Read the model definition and answer for the solid it produces. Units are mm, in the model's axes. A direction names the side the tool comes from. Coordinates: 2 decimals unless noted, no trailing zeros. Loops run counter-clockwise (first coordinate to the right, second up) from the corner with the lowest first, then second, coordinate; pieces in that order, holes last. Notation, with made-up numbers: (35, 66.25) -> (93, 66.25) arc R25 ccw to (93, 93.25) -> close; hole circle Ø3 at (35.5, 22.5). An arc over 180 degrees is marked (long way). Answer as a JSON object with one key per item and string values. Group by question number.
Q1. Determine the mould class of faces 1 (the flat face through (0, 0, -1.5)), 2 (the conical face through (17.49, 5.51, 0.34)), 3 (the cylindrical face through (0.526, 2.007, 77.669)) for opening direction X: released by +X, released by -X, zero draft, split by the parting line, or undercut.
Q2. Straight lines are drawn through the part: line 1 along Z through (x, y) = (-5, 4); line 2 along X through (y, z) = (2, 76); line 3 along Y through (x, z) = (0, 16.5). For each, find the intervals that lie inside material, in ascending order. Write a range as [from, to].
Q3. For faces 4 (the cylindrical face through (-0.867, -3.905, 67.649)), 5 (the flat face through (0, 2.5, 79)), 6 (the flat face through (8, -8, 0)), 7 (the flat face through (0, 1.5, 76)), determine the directions among +Z, -Z, +X, -X, +Y, -Y from which every point of the face is accessible in a straight line to the end or side of a thin tool.
Q4. The part is cut by section B-B on z = 23. Write down the section's boundary in (x, y), and give its area (3 significant figures).
Q5. Each of these flat-tipped pins is pushed along its axis until it touches: P1, Ø1, axis at y = -19.5, z = 37.5, coming from the +X side; P2, Ø4, axis at y = 7, z = 59, coming from the -X side; P3, Ø4, axis at x = -5.5, y = -13.5, coming from the -Z side; P4, Ø1.8, axis at x = 0.5, z = 76.5, coming from the +Y side. Where does it stop, or does it pass through?
Q6. The part is cut by section C-C on z = 76. Write down the section's boundary in (x, y).
Q7. The part is cut by section A-A on x = 0. Write down the section's boundary in (y, z).
from build123d import *

# Parameters (mm, degrees)
SKETCH_1_R          = 25
EXTRUDE_1_DEPTH     = 50
CHAMFER_1_SIZE      = 7
SKETCH_2_R          = 10
EXTRUDE_2_DEPTH     = 1.5
SKETCH_3_R          = 4
EXTRUDE_3_DEPTH     = 36
CUT_EXTRUDE_1_DEPTH = 18
SKETCH_5_R          = 1.75
CUT_EXTRUDE_2_DEPTH = 1
CHAMFER_2_SIZE      = 0.2


with BuildPart() as part:
    # 草图1 → 凸台-拉伸1 (new body)
    with BuildSketch(Plane.XY):
        Circle(SKETCH_1_R)
    extrude(amount=EXTRUDE_1_DEPTH)

    # 倒角1
    chamfer_1_edges = [part.edges().sort_by_distance(p)[0] for p in [
        (-25, 0, 0),
    ]]
    chamfer(chamfer_1_edges, length=CHAMFER_1_SIZE)

    # 草图2 → 凸台-拉伸2 (add)
    with BuildSketch(Plane(origin=(0, 0, 0), x_dir=(-1, 0, 0), z_dir=(0, 0, -1))):
        Circle(SKETCH_2_R)
    extrude(amount=EXTRUDE_2_DEPTH)

    # 草图3 → 凸台-拉伸3 (add)
    with BuildSketch(Plane.XY.offset(50)):
        Circle(SKETCH_3_R)
    extrude(amount=EXTRUDE_3_DEPTH)

    # 草图4 → 切除-拉伸1 (cut)
    with BuildSketch(Plane.XY.offset(86)):
        Polygon((-91.7895175, 2.5), (-3.122498999, 2.5), (3.122498999, 2.5), (91.7895175, 2.5), (91.7895175, 179.834037002), (-91.7895175, 179.834037002), align=None)
    extrude(amount=-CUT_EXTRUDE_1_DEPTH, mode=Mode.SUBTRACT)

    # 草图5 → 切除-拉伸2 (cut)
    with BuildSketch(Plane(origin=(0, 2.5, 0), x_dir=(1, 0, 0), z_dir=(0, 1, 0))):
        with Locations(Location((0, -76, 0), (0, 0, 270))):
            Circle(SKETCH_5_R)
    extrude(amount=-CUT_EXTRUDE_2_DEPTH, mode=Mode.SUBTRACT)

    # 倒角2
    chamfer_2_edges = [part.edges().sort_by_distance(p)[0] for p in [
        (-1.324764885, -3.774254628, 86),
        (0, 2.5, 86),
    ]]
    chamfer(chamfer_2_edges, length=CHAMFER_2_SIZE)


solid = part.part
Final values:
{
 "1": {"face 1": "zero draft", "face 2": "split by the parting line", "face 3": "undercut"},
 "2": {"line 1": "z = [-1.5, 50]", "line 2": "x = [-3.46, -1.75], [1.75, 3.46]", "line 3": "y = [-25, 25]"},
 "3": {"face 4": "+Z", "face 5": "+Z, +X, -X, +Y", "face 6": "-Z", "face 7": "+Y"},
 "4": {"outline": "circle Ø50 at (0, 0)", "area": "1,960 mm2"},
 "5": {"P1": "stops at x = 16.25", "P2": "passes through", "P3": "stops at z = 0", "P4": "stops at y = 1.5"},
 "6": {"outline": "(-3.12, 2.5) arc R4 ccw (long way) to (3.12, 2.5) -> (1.75, 2.5) -> (1.75, 1.5) -> (-1.75, 1.5) -> (-1.75, 2.5) -> close"},
 "7": {"outline": "(-25, 7) -> (-18, 0) -> (-10, 0) -> (-10, -1.5) -> (10, -1.5) -> (10, 0) -> (18, 0) -> (25, 7) -> (25, 50) -> (4, 50) -> (4, 68) -> (2.5, 68) -> (2.5, 74.25) -> (1.5, 74.25) -> (1.5, 77.75) -> (2.5, 77.75) -> (2.5, 85.8) -> (2.3, 86) -> (-3.8, 86) -> (-4, 85.8) -> (-4, 50) -> (-25, 50) -> close"}
}
